Geometry: final body of the model. Coordinates: model frame, mm. Face numbers are marked on the shaded views. A direction names the side the tool comes from. Give positions to 0.01 mm unless a question says otherwise; leave off trailing zeros. Loops run counter-clockwise (first coordinate to the right, second up) from the corner with the lowest first, then second, coordinate; pieces in that order, holes last. Notation, with made-up numbers: (55, 20.25) - (103, 20.25) arc R24 cw to (103, 54.25) - close; hole circle Ø2 at (-13.75, -26.5). An arc over 180 degrees is marked (long way). Use one line per item in the form item = value.
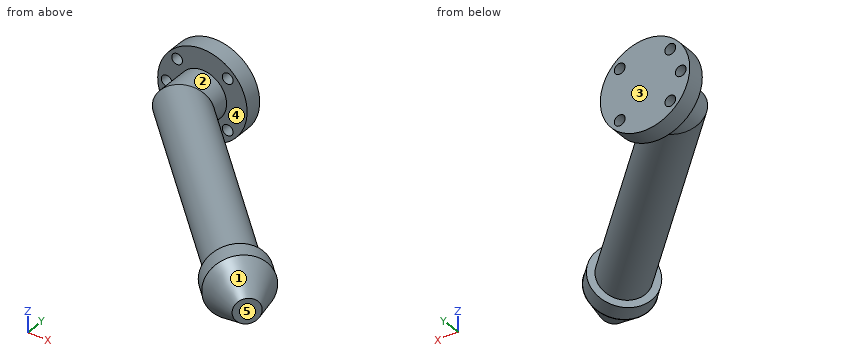
Autodesk Inventor part; units mm, degrees
ref_plane "YZ Plane" through (0, 0, 0) normal (1, 0, 0) x (0, 1, 0)
ref_plane "XZ Plane" through (0, 0, 0) normal (0, 1, 0) x (-1, 0, 0)
ref_plane "XY Plane" through (0, 0, 0) normal (0, 0, 1) x (1, 0, 0)
sketch "Boceto1" plane through (0, 0, 0) normal (0, 1, 0) x (-1, 0, 0)
  circle A0 centre (0, 0) radius 25
  circle A1 centre (0, 0) radius 20
  line L0 (0, 0) -> (25, 0)
  line L1 (0, 0) -> (17.67767, -17.67767)
  line L2 (0, 0) -> (25, 0) construction
  line L3 (0, 0) -> (17.67767, 17.67767)
  line L4 (0, 0) -> (25, 0) construction
  line L5 (0, 0) -> (-17.67767, -17.67767)
  line L6 (0, 0) -> (-17.67767, 17.67767)
  circle A2 centre (20, 0) radius 3
  circle A3 centre (14.142136, -14.142136) radius 3
  circle A4 centre (14.142136, 14.142136) radius 3
  circle A5 centre (-14.142136, 14.142136) radius 3
  circle A6 centre (-14.142136, -14.142136) radius 3
  point P0 (16.098382, 11.867691)
  point P1 (11.867691, 16.098382)
  dimension "d0" = 50
  dimension "d1" = 40
  dimension "d2" = 45
  dimension "d3" = 45
  dimension "d4" = 6
  dimension "d5" = 6
  dimension "d6" = 6
  dimension "d7" = 6
  dimension "d8" = 6
extrude "Extrusión1" add sketch "Boceto1" along normal blind 10 contours L0 A2 A1 A4 L3 A0 | A0 L1 A3 A1 A2 L0 | L3 A4 A1 A5 L6 A0 | A0 L5 A6 A1 A3 L1 | L6 A5 A1 A6 L5 A0 | A2 L0 L3 A4 A1 | A1 A3 L1 L0 A2 | A4 L3 L6 A5 A1 | A1 A6 L5 L1 A3 | A5 L6 L5 A6 A1
thread "Rosca1"
thread "Rosca2"
thread "Rosca3"
thread "Rosca4"
sketch "Boceto7" plane through (0, 0, 0) normal (0, 0, 1) x (1, 0, 0)
  line L0 (0, 0) -> (0, -15)
  line L1 (0, -15) -> (98.994949, -113.994949)
  dimension "d31" = 15
  dimension "d32" = 140
  dimension "d33" = 135
sketch "Boceto8" plane through (0, 0, 0) normal (0, -1, 0) x (1, 0, 0)
  circle A0 centre (0, 0) radius 13.5
  dimension "d34" = 27
sweep "Barrido1" add profiles "Boceto8" path "Boceto7"
sketch "Boceto13" plane through (0, 0, 0) normal (0, 0, 1) x (1, 0, 0)
  line L0 (0, 0) -> (0, -15)
  line L1 (0, -15) -> (120.208153, -135.208153)
  dimension "d48" = 170
  dimension "d49" = 135
sketch "Boceto14" plane through (98.994949, -113.994949, 0) normal (0.7071068, -0.7071068, 0) x (-0.7071068, -0.7071068, 0)
  ellipse E0 centre (-17.67767, 0) end of major axis (-17.67767, -25) minor radius 17.67767
  circle A0 centre (0, 0) radius 17.5
  point P0 (-10.606602, 0)
  dimension "d50" = 35
extrude "Extrusión9" add sketch "Boceto14" along normal blind 10 contours A0 E0 | E0 A0 picked at (-5.916701, -1.209366) picked at (5.555683, -1.849173)
ref_plane "Plano de trabajo1" through (120.208153, -135.208153, 0) normal (0.7071068, -0.7071068, 0) x (0.7071068, 0.7071068, 0)
sketch "Boceto16" plane through (120.208153, -135.208153, 0) normal (0.7071068, -0.7071068, 0) x (0.7071068, 0.7071068, 0)
  ellipse E0 centre (17.67767, 0) end of major axis (17.67767, 25) minor radius 17.67767
  circle A0 centre (0, 0) radius 7
  point P0 (10.606602, 0)
  dimension "d58" = 14
sketch "Boceto16 outline for Extrusión10" plane through (120.208153, -135.208153, 0) normal (0.7071068, -0.7071068, 0) x (0.7071068, 0.7071068, 0)
  circle A0 centre (0, 0) radius 7
extrude "Extrusión10" add sketch "Boceto16 outline for Extrusión10" against normal blind 20 draft 28
properties part number "Herramienta total"
(1) Pin query (flat end, axial travel): P1, Ø10, axis at x = 74, y = -104, coming from the +Z side; P2, Ø3, axis at y = -100.5, z = 6.5, coming from the +X side; P3, Ø2, axis at x = 27.5, z = -8, coming from the -Y side. Return the tip coordinate at first contact, or that it passes through.
Solution:
P1 = 12.28
P2 = 104.08
P3 = -59.27
(2) Pull-direction query (Y, two-part tool) for the marked faces 1, 2 and 3; classes: released by +Y, released by -Y, zero draft, split by the parting line, or undercut.
Solution:
face_1 = split by the parting line
face_2 = undercut
face_3 = released by +Y
(3) Material intervals for L1, parallel to Z at x = -17.5, y = 0.5; L2, parallel to Z at x = -20, y = 3.75; L3, parallel to Y at x = 12, z = -20, sorted ascending. Write a range as from..to.
Solution:
L1 = -17.85..-1.66, 1.66..17.85
L2 = -15..-3, 3..15
L3 = 0..10
(4) Cut plane B-B (z = 0). Return the cut outline in (x, y).
Solution:
outline = (-25, 0) - (-23, 0) - (-23, 10) - (-25, 10) - close; (-17, 0) - (-13.5, 0) - (-13.5, -20.59) - (89.45, -123.54) - (86.62, -126.37) - (93.69, -133.44) - (93.6, -133.54) - (115.26, -140.16) - (125.16, -130.26) - (118.54, -108.6) - (118.44, -108.69) - (111.37, -101.62) - (108.54, -104.45) - (13.5, -9.41) - (13.5, 0) - (25, 0) - (25, 10) - (-17, 10) - close
(5) Access query for the marked faces 4 and 5. Directions: +Z, -Z, +X, -X, +Y, -Y. A direction counts if a zero-diameter tool reaches every point of the face in a straight line with its end or side. Return the directions, or none.
Solution:
face_4 = none
face_5 = +Z, -Z, +X, -Y
(6) Cut plane A-A (x = -20). Return the cut outline in (y, z).
Solution:
outline = (0, -15) - (10, -15) - (10, -3) - (0, -3) - close; (0, 3) - (10, 3) - (10, 15) - (0, 15) - close
